```python
from build123d import *

# Parameters (mm, degrees)
EXTRUDE_1_DEPTH = 4


with BuildPart() as part:
    # Эскиз1 → Бобышка-Вытянуть1 (new body)
    with BuildSketch(Plane(origin=(0, 0, 0), x_dir=(0, 0, -1), z_dir=(1, 0, 0))):
        with BuildLine():
            Line((-1, 24), (1, 24))
            Line((1, 24), (1.920801391, 19.907549372))
            ThreePointArc((1.920801391, 19.907549372), (6.180339887, 19.021130326), (10.147402962, 17.234564489))
            Line((10.147402962, 17.234564489), (13.297829061, 20.004193117))
            Line((13.297829061, 20.004193117), (14.915863049, 18.828622613))
            Line((14.915863049, 18.828622613), (13.255324899, 14.976527028))
            ThreePointArc((13.255324899, 14.976527028), (16.180339887, 11.755705046), (18.339644281, 7.978561752))
            Line((18.339644281, 7.978561752), (22.516339397, 8.367464381))
            Line((22.516339397, 8.367464381), (23.134373385, 6.465351349))
            Line((23.134373385, 6.465351349), (19.526764827, 4.324980393))
            ThreePointArc((19.526764827, 4.324980393), (20, 0), (19.526764827, -4.324980393))
            Line((19.526764827, -4.324980393), (23.134373385, -6.465351349))
            Line((23.134373385, -6.465351349), (22.516339397, -8.367464381))
            Line((22.516339397, -8.367464381), (18.339644281, -7.978561752))
            ThreePointArc((18.339644281, -7.978561752), (16.180339887, -11.755705046), (13.255324899, -14.976527028))
            Line((13.255324899, -14.976527028), (14.915863049, -18.828622613))
            Line((14.915863049, -18.828622613), (13.297829061, -20.004193117))
            Line((13.297829061, -20.004193117), (10.147402962, -17.234564489))
            ThreePointArc((10.147402962, -17.234564489), (6.180339887, -19.021130326), (1.920801391, -19.907549372))
            Line((1.920801391, -19.907549372), (1, -24))
            Line((1, -24), (-1, -24))
            Line((-1, -24), (-1.920801391, -19.907549372))
            ThreePointArc((-1.920801391, -19.907549372), (-6.180339887, -19.021130326), (-10.147402962, -17.234564489))
            Line((-10.147402962, -17.234564489), (-13.297829061, -20.004193117))
            Line((-13.297829061, -20.004193117), (-14.915863049, -18.828622613))
            Line((-14.915863049, -18.828622613), (-13.255324899, -14.976527028))
            ThreePointArc((-13.255324899, -14.976527028), (-16.180339887, -11.755705046), (-18.339644281, -7.978561752))
            Line((-18.339644281, -7.978561752), (-22.516339397, -8.367464381))
            Line((-22.516339397, -8.367464381), (-23.134373385, -6.465351349))
            Line((-23.134373385, -6.465351349), (-19.526764827, -4.324980393))
            ThreePointArc((-19.526764827, -4.324980393), (-20, 0), (-19.526764827, 4.324980393))
            Line((-19.526764827, 4.324980393), (-23.134373385, 6.465351349))
            Line((-23.134373385, 6.465351349), (-22.516339397, 8.367464381))
            Line((-22.516339397, 8.367464381), (-18.339644281, 7.978561752))
            ThreePointArc((-18.339644281, 7.978561752), (-16.180339887, 11.755705046), (-13.255324899, 14.976527028))
            Line((-13.255324899, 14.976527028), (-14.915863049, 18.828622613))
            Line((-14.915863049, 18.828622613), (-13.297829061, 20.004193117))
            Line((-13.297829061, 20.004193117), (-10.147402962, 17.234564489))
            ThreePointArc((-10.147402962, 17.234564489), (-6.180339887, 19.021130326), (-1.920801391, 19.907549372))
            Line((-1.920801391, 19.907549372), (-1, 24))
        make_face()
    extrude(amount=EXTRUDE_1_DEPTH)


solid = part.part
```
Geometry: final body of the model. Coordinates: model frame, mm. A direction names the side the tool comes from. Round coordinates to 2 decimals unless told otherwise and drop trailing zeros. Order: outer loops, then holes, each group sorted by start corner. A loop starts at its lowest first (then second) coordinate and runs counter-clockwise, first axis right, second up. Notation, with made-up numbers: (75.5, 60) -> (122.5, 60) arc R27 cw to (122.5, 96) -> close; hole circle Ø11 at (8, 69). An arc over 180 degrees is marked (long way). Use one line per item in the form item = value. Start each with the question number.
1. Cut plane A-A (y = 0). Return the cut outline in (x, z).
2. Cut plane B-B (z = 8.5). Return the cut outline in (x, y), then the cut area to 3 significant figures.
3. Reachability of faces 1 (the face through (2, 0, -20)), 2 (the face through (1.97, -19, -6.24)), 3 (the face through (2, 24, 0)), 4 (the face through (1.972, -16.93, 14.097)), 5 (the face through (1.97, 19, 6.24)) from +Z, -Z, +X, -X, +Y, -Y: full face, straight path, thin tool, end or side. Return the list, or none.
4. Pin query (flat end, axial travel): pin 1 Ø2 at (x, z) = (2.5, 7) entering from +Y. Return the tip coordinate at first contact, or that it passes through.
5. Draft query along Y for faces 6 (the face through (1.972, 19.408, 14.118)), 7 (the face through (1.972, -5.38, -21.305)), 8 (the face through (2, -18.6, -11.7)). Return one class per face: pulls with the +Y half, pulls with the -Y half, needs draft (parallel to the pull), parting line crosses it, or undercut.
6. Line query: probe 1 along Z at (x, y) = (2.5, 18); probe 2 along Z at (x, y) = (2.4, 0); probe 3 along Y at (x, z) = (1.3, -2). Output: solid intervals per line, ascending.
Solution:
q1.outline = (0, -20) -> (4, -20) -> (4, 20) -> (0, 20) -> close
q2.outline = (0, -18.1) -> (4, -18.1) -> (4, 18.1) -> (0, 18.1) -> close
q2.area = 145 mm^2
q3.face_1 = -Z, +X, -X
q3.face_2 = +X, -X, -Y
q3.face_3 = +Z, -Z, +X, -X, +Y
q3.face_4 = +Z, +X, -X
q3.face_5 = +X, -X, +Y
q4.pin_1 = 19.08
q5.face_6 = pulls with the +Y half
q5.face_7 = undercut
q5.face_8 = pulls with the -Y half
q6.probe_1 = -14.56 to -11.02, -8.72 to 8.72, 11.02 to 14.56
q6.probe_2 = -20 to 20
q6.probe_3 = -19.9 to 19.9
